Check sheet for the drawn part. Datum: minimum x, y, z corner. Units: mm. A direction names the side the tool comes from. Round coordinates to 2 decimals unless told otherwise and drop trailing zeros. Write each loop counter-clockwise with the first axis right and the second up, starting at its lowest first coordinate (ties: lowest second). Pieces come first, ordered by that corner, then holes. Notation, with made-up numbers: (-13, 61) -> (-8, 61) arc R20 ccw to (-8, 99) -> close; hole circle Ø8 at (-16, -34.75). An arc over 180 degrees is marked (long way). Use a Markdown table: item, result.
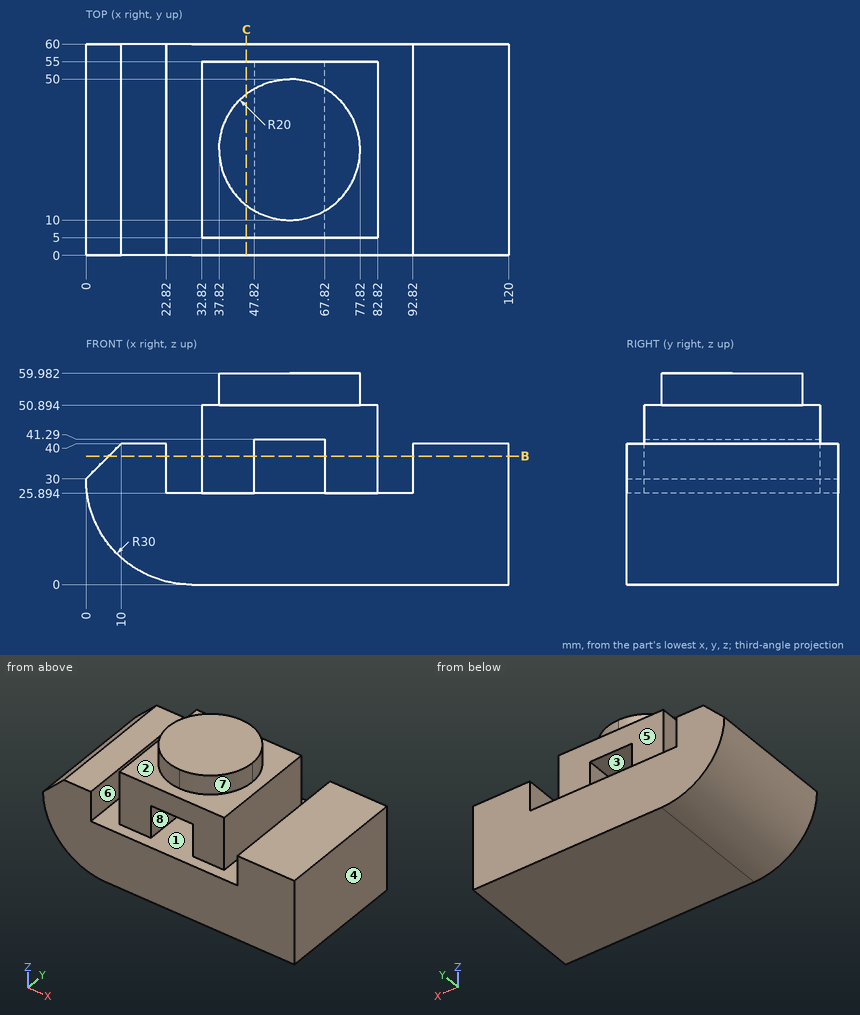
(1) Section check B-B on z = 36.5. Record the cut outline in (x, y).
A:
| item | result |
|---|---|
| outline | (6.5, 0) -> (22.82, 0) -> (22.82, 60) -> (6.5, 60) -> close; (32.82, 5) -> (47.82, 5) -> (47.82, 55) -> (32.82, 55) -> close; (67.82, 5) -> (82.82, 5) -> (82.82, 55) -> (67.82, 55) -> close; (92.82, 0) -> (120, 0) -> (120, 60) -> (92.82, 60) -> close |
(2) Gauge pin test, flat ends, axial feed: pin 1 Ø1 at (y, z) = (45, 21.5) entering from -X; pin 2 Ø12 at (x, y) = (93.5, 16.5) entering from +Z; pin 3 Ø1.5 at (x, z) = (54, 50) entering from +Y. Record the tip position at first contact, or that the pin passes through.
A:
| item | result |
|---|---|
| pin 1 | stops at x = 1.09 |
| pin 2 | stops at z = 40 |
| pin 3 | stops at y = 55 |
(3) Thickness scan on line 1 (Z direction, x = 65, y = 26.5); line 2 (X direction, y = 24.5, z = 33.5); line 3 (X direction, y = 49.5, z = 38.5). Record the ranges inside material, lowest first.
A:
| item | result |
|---|---|
| line 1 | z = 0 to 25.89, 41.29 to 59.98 |
| line 2 | x = 3.5 to 22.82, 32.82 to 47.82, 67.82 to 82.82, 92.82 to 120 |
| line 3 | x = 8.5 to 22.82, 32.82 to 47.82, 67.82 to 82.82, 92.82 to 120 |
(4) Access from +Z, -Z, +X, -X, +Y, -Y to the whole of each face (thin tool, end or side, straight path). Record for the marked faces 5, 6, 7 and 8.
A:
| item | result |
|---|---|
| face 5 | +Z, +Y |
| face 6 | +Z, +Y, -Y |
| face 7 | +Z, +X, -Y |
| face 8 | +Y, -Y |
(5) Section check C-C on x = 45.5. Record the cut outline in (y, z) (1 decimal), plus the area to 3 significant figures.
A:
| item | result |
|---|---|
| outline | (0, 0) -> (60, 0) -> (60, 25.9) -> (55, 25.9) -> (55, 50.9) -> (45.8, 50.9) -> (45.8, 60) -> (14.2, 60) -> (14.2, 50.9) -> (5, 50.9) -> (5, 25.9) -> (0, 25.9) -> close |
| area | 3,090 mm2 |
(6) Release check for a two-part mould opening along X. For the marked faces 1, 2, 3 and 4 record: +X half, -X half, draft (parallel to the pull), parting line (faces both ways), or undercut.
A:
| item | result |
|---|---|
| face 1 | undercut |
| face 2 | draft |
| face 3 | undercut |
| face 4 | +X half |
